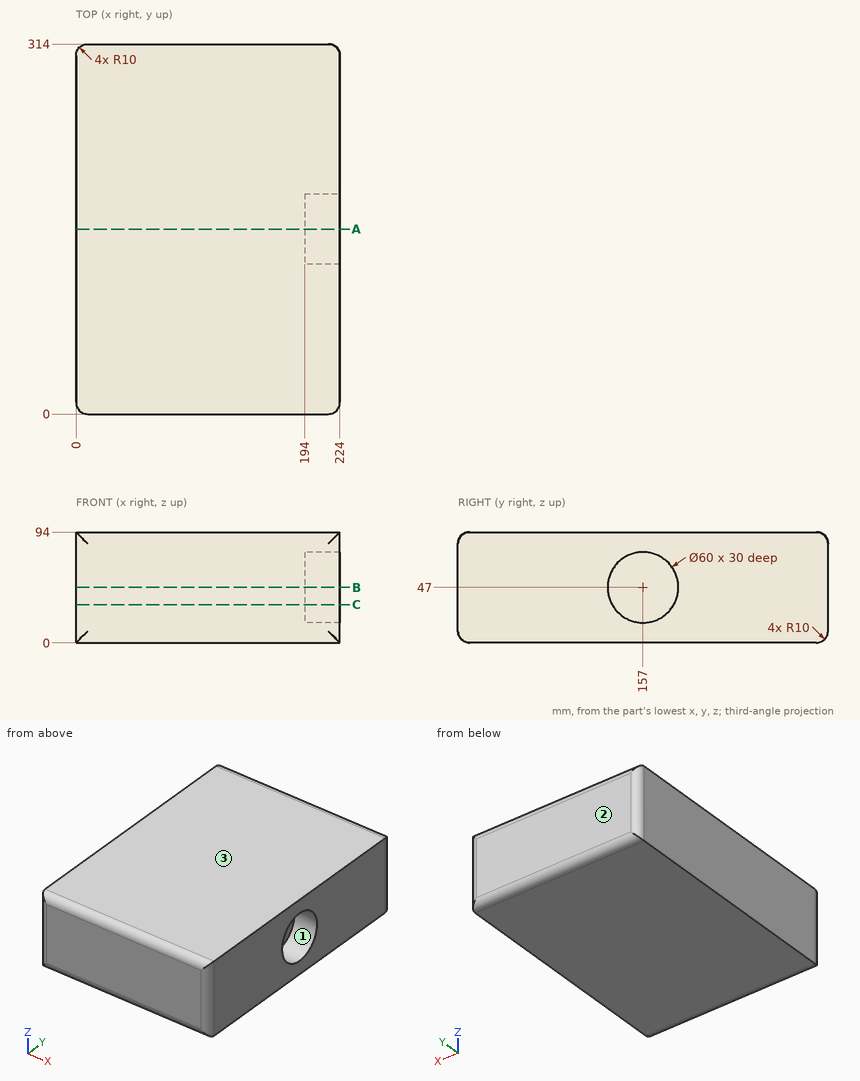
Geometry check sheet. Reference: drawing and pictorial views, mm from the part's lowest x, y, z. Give positions to 0.01 mm unless a question says otherwise; leave off trailing zeros. Write each loop counter-clockwise with the first axis right and the second up, starting at its lowest first coordinate (ties: lowest second). Pieces come first, ordered by that corner, then holes.
Item 1: Cross-section at A-A (y = 157). Enter the section's corners in (x, z).
Item 2: Draft check along Y on the marked faces 1, 2 and 3. Enter one of: released by +Y, released by -Y, zero draft, split by the parting line, or undercut.
Item 3: Gauge pin test, flat end, axial feed: pin 1 (3 mm diameter, centred on y = 159, z = 60.5, fed in from +X). Record the tip position at first contact, or that the pin passes through.
Item 4: Cross-section at C-C (z = 32.5). Enter the section's corners in (x, y), and give its area (3 significant figures).
Item 5: Scan lines: L1, parallel to Z at x = 206, y = 157; L2, parallel to X at y = 173, z = 44; L3, parallel to Y at x = 199, z = 62. Record each from-to range of solid material in increasing order.
Item 6: Cross-section at B-B (z = 47). Enter the section's corners in (x, y).
Report:
1. outline: (0, 0) - (224, 0) - (224, 17) - (194, 17) - (194, 77) - (224, 77) - (224, 94) - (0, 94) - close
2. face 1: undercut
2. face 2: released by +Y
2. face 3: zero draft
3. pin 1: stops at x = 194
4. outline: (0, 10) arc R10 ccw to (10, 0) - (214, 0) arc R10 ccw to (224, 10) - (224, 130.74) - (194, 130.74) - (194, 183.26) - (224, 183.26) - (224, 304) arc R10 ccw to (214, 314) - (10, 314) arc R10 ccw to (0, 304) - close
4. area: 68,700 mm2
5. L1: z = 0 to 17, 77 to 94
5. L2: x = 0 to 194
5. L3: y = 0 to 131.02, 182.98 to 314
6. outline: (0, 10) arc R10 ccw to (10, 0) - (214, 0) arc R10 ccw to (224, 10) - (224, 127) - (194, 127) - (194, 187) - (224, 187) - (224, 304) arc R10 ccw to (214, 314) - (10, 314) arc R10 ccw to (0, 304) - close
